```python
from build123d import *

# Parameters (mm, degrees)
SKETCH2_W           = 115
SKETCH2_H           = 21.5
BOSS_EXTRUDE1_DEPTH = 35
BOSS_EXTRUDE2_DEPTH = 3
SKETCH8_W           = 105
SKETCH8_H           = 11.5
CUT_EXTRUDE2_DEPTH  = 30
SKETCH9_R           = 1.46
CUT_EXTRUDE3_DEPTH  = 33
SKETCH10_W          = 15
SKETCH10_H          = 8.5
CUT_EXTRUDE4_DEPTH  = 88


with BuildPart() as part:
    # Sketch2 → Boss-Extrude1 (new body)
    with BuildSketch(Plane.XY):
        with Locations((9.785277127, -0.97863388)):
            Rectangle(SKETCH2_W, SKETCH2_H)
    extrude(amount=BOSS_EXTRUDE1_DEPTH)

    # Sketch7 → Boss-Extrude2 (add)
    with BuildSketch(Plane.XY):
        with BuildLine():
            Line((-47.714722873, 19.77136612), (67.285277127, 19.77136612))
            ThreePointArc((67.285277127, 19.77136612), (74.356344939, 16.842433932), (77.285277127, 9.77136612))
            Line((77.285277127, 9.77136612), (77.285277127, -11.72863388))
            ThreePointArc((77.285277127, -11.72863388), (74.356344939, -18.799701692), (67.285277127, -21.72863388))
            Line((67.285277127, -21.72863388), (-47.714722873, -21.72863388))
            ThreePointArc((-47.714722873, -21.72863388), (-54.785790685, -18.799701692), (-57.714722873, -11.72863388))
            Line((-57.714722873, -11.72863388), (-57.714722873, 9.77136612))
            ThreePointArc((-57.714722873, 9.77136612), (-54.785790685, 16.842433932), (-47.714722873, 19.77136612))
        make_face()
    extrude(amount=BOSS_EXTRUDE2_DEPTH)

    # Sketch8 → Cut-Extrude2 (cut)
    with BuildSketch(Plane.XY):
        with Locations((9.785277127, -0.97863388)):
            Rectangle(SKETCH8_W, SKETCH8_H)
    extrude(amount=CUT_EXTRUDE2_DEPTH, mode=Mode.SUBTRACT)

    # Sketch9 → Cut-Extrude3 (cut)
    with BuildSketch(Plane.XY):
        with Locations((38.285277127, 14.68536612)):
            Circle(SKETCH9_R)
        with Locations((-18.714722873, 15.00736612)):
            Circle(SKETCH9_R)
        with Locations((-18.714722873, -16.34263388)):
            Circle(SKETCH9_R)
        with Locations((38.285277127, -16.66463388)):
            Circle(SKETCH9_R)
    extrude(amount=CUT_EXTRUDE3_DEPTH, mode=Mode.SUBTRACT)

    # Sketch10 → Cut-Extrude4 (cut)
    with BuildSketch(Plane(origin=(0, 0, 0), x_dir=(0, 0, -1), z_dir=(1, 0, 0))):
        with Locations((-19, -0.97863388)):
            Rectangle(SKETCH10_W, SKETCH10_H)
    extrude(amount=-CUT_EXTRUDE4_DEPTH, mode=Mode.SUBTRACT)


solid = part.part
```
Part model, mm, in its own coordinate system. A direction names the side the tool comes from. Round coordinates to 2 decimals unless told otherwise and drop trailing zeros. Write each loop counter-clockwise with the first axis right and the second up, starting at its lowest first coordinate (ties: lowest second). Pieces come first, ordered by that corner, then holes. Notation, with made-up numbers: (88.25, 66) -> (129.25, 66) arc R24 ccw to (129.25, 100) -> close; hole circle Ø4 at (0.25, -18.75). An arc over 180 degrees is marked (long way). Return JSON: item names as keys, results as strings. Group by question number.
Q1. Pin check, flat tips, straight feed: pin 1 (3 mm diameter, centred on x = -26.5, y = -1.5, fed in from -Z); pin 2 (3.5 mm diameter, centred on x = 38.29, y = 14.69, fed in from +Z); pin 3 (4 mm diameter, centred on y = -13.5, z = 19.5, fed in from +X). Stop position of each tip, or through.
Q2. Saw through at C-C on x = 49. Write the cut outline in (y, z).
Q3. Probe L1, parallel to Y at x = -12, z = 29.5; L2, parallel to Z at x = -43.5, y = 1.5; L3, parallel to X at y = -3, z = 29. List the from-to ranges inside material, lowest first. Write a range as [from, to].
Q4. Which spindle directions (+Z, -Z, +X, -X, +Y, -Y) get a long thin tool onto all of the face, cutting with end or side? Do faces 4 (the flat face through (11, -21.729, 1)), 5 (the flat face through (-45, 3.271, 19)), 6 (the flat face through (62.285, -1, 15)). Say none if no direction does.
Q5. Saw through at B-B on z = 28. Write the cut outline in (x, y).
Q6. Saw through at D-D on y = 7.5. Write the cut outline in (x, z).
Q7. Saw through at A-A on y = 0.5. Write the cut outline in (x, z), plus the area to 3 significant figures.
Q8. Mould opens along Z. For faces 1 (the cylindrical face through (74.3, 16.9, 1.5)), 2 (the flat face through (9, -1, 30)), 3 (the flat face through (-45, -1, 26.5)) say: pulls with the +Z half, pulls with the -Z half, needs draft (parallel to the pull), parting line crosses it, or undercut.
Answer:
{
 "1": {"pin 1": "z = 30", "pin 2": "z = 3", "pin 3": "x = 67.29"},
 "2": {"outline": "(-21.73, 0) -> (-6.73, 0) -> (-6.73, 30) -> (4.77, 30) -> (4.77, 0) -> (19.77, 0) -> (19.77, 3) -> (9.77, 3) -> (9.77, 35) -> (-11.73, 35) -> (-11.73, 3) -> (-21.73, 3) -> close"},
 "3": {"L1": "[-11.73, -6.73], [4.77, 9.77]", "L2": "[0, 11.5], [26.5, 35]", "L3": "[-47.71, -42.71], [62.29, 67.29]"},
 "4": {"face 4": "+Z, -Z, +X, -X, -Y", "face 5": "-X", "face 6": "-Z"},
 "5": {"outline": "(-47.71, -11.73) -> (67.29, -11.73) -> (67.29, 9.77) -> (-47.71, 9.77) -> close; hole (-42.71, -6.73) -> (62.29, -6.73) -> (62.29, 4.77) -> (-42.71, 4.77) -> close"},
 "6": {"outline": "(-57.71, 0) -> (77.29, 0) -> (77.29, 3) -> (67.29, 3) -> (67.29, 35) -> (-47.71, 35) -> (-47.71, 3) -> (-57.71, 3) -> close"},
 "7": {"outline": "(-57.71, 0) -> (-42.71, 0) -> (-42.71, 11.5) -> (-47.71, 11.5) -> (-47.71, 3) -> (-57.71, 3) -> close; (-47.71, 26.5) -> (-42.71, 26.5) -> (-42.71, 30) -> (62.29, 30) -> (62.29, 0) -> (77.29, 0) -> (77.29, 3) -> (67.29, 3) -> (67.29, 35) -> (-47.71, 35) -> close", "area": "860 mm2"},
 "8": {"face 1": "needs draft", "face 2": "pulls with the -Z half", "face 3": "undercut"}
}
